Here's the drawing with two shaded views (mm, measured from the low corner). I have some questions. Coordinates: 2 decimals unless noted, no trailing zeros. Order: outer loops, then holes, each group sorted by start corner. A loop starts at its lowest first (then second) coordinate and runs counter-clockwise, first axis right, second up. Notation, with made-up numbers: (-21, 70.25) -> (6, 70.25) arc R4 cw to (6, 76.25) -> close; hole circle Ø3 at (-33.5, 23). An arc over 180 degrees is marked (long way). Answer as a JSON object with one key per item and string values. Group by question number.
(1) For pin 1 (1.6 mm diameter, centred on y = 67, z = 1, fed in from -X) (3 decimals); pin 2 (7.5 mm diameter, centred on x = 117.475, y = 101.6, fed in from -Z); pin 3 (1 mm diameter, centred on y = 129.5, z = 1, fed in from +X) (3 decimals), each with a flat end and sliding along its axis, tell me the tip position at first contact or that it passes through.
(2) I need wall thicknesses on line 1 (X direction, y = 125.5, z = 1.1) (3 decimals). Which ranges of the line are inside material? Lowest first, please.
(3) If we mould it in two halves opening along Z, with no side actions, what happens to the marked faces 1 and 2? For each: pulls with the +Z half, pulls with the -Z half, needs draft (parallel to the pull), parting line crosses it, or undercut.
(4) I want a section at A-A, the plane y = 101.6. List the corners of the cut face in (x, z) for me (1 decimal).
(5) I want a section at C-C, the plane y = 165. List the corners of the cut face in (x, z) for me (3 decimals), plus the area to 3 significant figures.
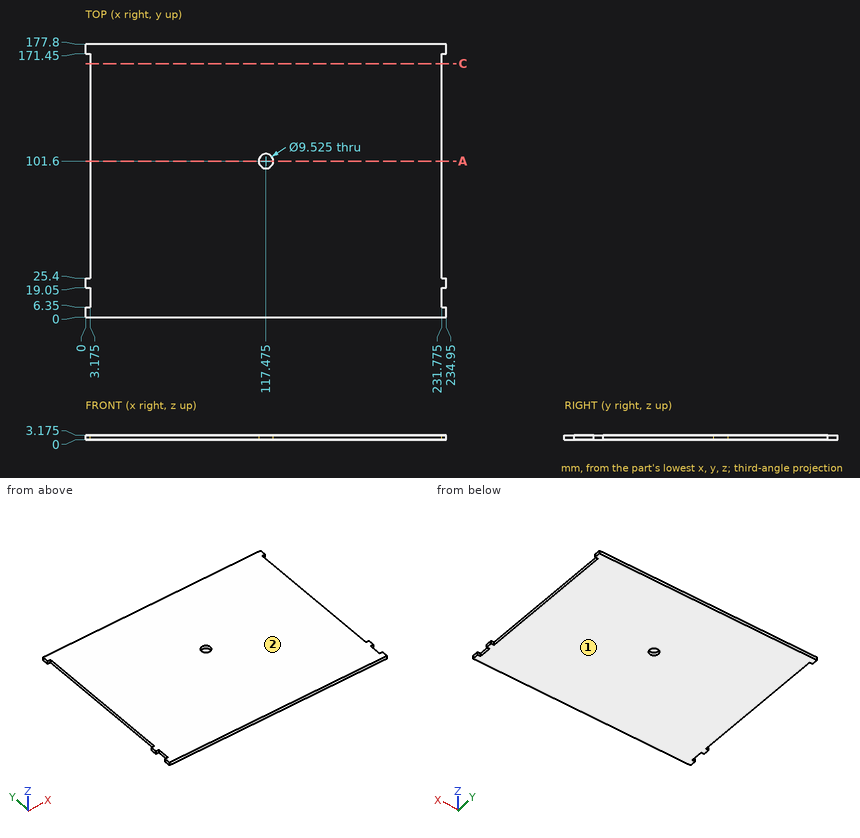
Computed values:
{
 "1": {"pin 1": "stops at x = 3.175", "pin 2": "passes through", "pin 3": "stops at x = 231.775"},
 "2": {"line 1": "x = 3.175 to 231.775"},
 "3": {"face 1": "pulls with the -Z half", "face 2": "pulls with the +Z half"},
 "4": {"outline": "(3.2, 0) -> (112.7, 0) -> (112.7, 3.2) -> (3.2, 3.2) -> close; (122.2, 0) -> (231.8, 0) -> (231.8, 3.2) -> (122.2, 3.2) -> close"},
 "5": {"outline": "(3.175, 0) -> (231.775, 0) -> (231.775, 3.175) -> (3.175, 3.175) -> close", "area": "726 mm2"}
}
